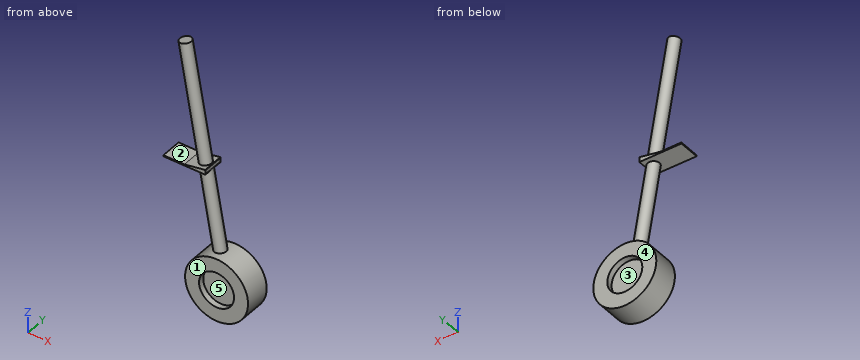
from build123d import *

# Parameters (mm, degrees)
F0_W      = 180
F0_H      = 90
F1_DEPTH  = 5
F3_DEPTH  = 90
F4_R      = 25
F5_DEPTH  = 495
F6_DEPTH  = 500
F9_R      = 135
F10_DEPTH = 55
F11_R     = 75
F12_DEPTH = 25
F13_R     = 75
F14_DEPTH = 25


with BuildPart() as f1:
    # F0 (on Top) → F1 (new body)
    with BuildSketch(Plane.XY):
        Rectangle(F0_W, F0_H)
    extrude(amount=F1_DEPTH)

    # F2 (on face) → F3 (join)
    with BuildSketch(Plane.XZ.offset(45)):
        Polygon((88.6326977711, 20.62833599), (0, 5), (28.4956841358, 5), (89.5009386594, 15.704297225), align=None)
        Polygon((89.5009386594, 15.704297225), (28.4956841358, 5), (90, 5), align=None)
    extrude(amount=-F3_DEPTH)

    # F4 (on face) → F5 (join)
    with BuildSketch(Plane(origin=(-0.8550503583, 0, 4.849231552), x_dir=(0.984807753, 0, 0.1736481777), z_dir=(-0.1736481777, 0, 0.984807753))):
        with Locations((60.8682408883, 0)):
            Circle(F4_R)
    extrude(amount=-F5_DEPTH)

    # F4 (on face) → F6 (join)
    with BuildSketch(Plane(origin=(-0.8550503583, 0, 4.849231552), x_dir=(0.984807753, 0, 0.1736481777), z_dir=(-0.1736481777, 0, 0.984807753))):
        with Locations((60.8682408883, 0)):
            Circle(F4_R)
    extrude(amount=F6_DEPTH)

    # F9 (on line) → F10 (join, symmetric)
    with BuildSketch(Plane(origin=(0, 0, 0), x_dir=(-1, 0, 0), z_dir=(0, 1, 0))):
        with Locations((-145.0443131259, -472.060947081)):
            Circle(F9_R)
    extrude(amount=F10_DEPTH, both=True)

    # F11 (on face) → F12 (cut)
    with BuildSketch(Plane.XZ.offset(55)):
        with Locations((145.0443131259, -472.060947081)):
            Circle(F11_R)
    extrude(amount=-F12_DEPTH, mode=Mode.SUBTRACT)

    # F13 (on face) → F14 (cut)
    with BuildSketch(Plane(origin=(0, 55, 0), x_dir=(-1, 0, 0), z_dir=(0, 1, 0))):
        with Locations((-145.0443131259, -472.060947081)):
            Circle(F13_R)
    extrude(amount=-F14_DEPTH, mode=Mode.SUBTRACT)


solid = f1.part
The model under review builds one solid part; all positions refer to its coordinate system, in mm. Face numbers are marked on the shaded views. A direction names the side the tool comes from. Round coordinates to 2 decimals unless told otherwise and drop trailing zeros. Write each loop counter-clockwise with the first axis right and the second up, starting at its lowest first coordinate (ties: lowest second). Pieces come first, ordered by that corner, then holes. Notation, with made-up numbers: (-10, -37.5) -> (-1, -37.5) arc R27 cw to (-1, -10.5) -> close; hole circle Ø9 at (-8.5, -34.75). An arc over 180 degrees is marked (long way). Answer as a JSON object with one key per item and string values.
1. We need section C-C on x = 204.5. State the section outline as (y, z) points, and give its area (3 significant figures).
Results found:
{"outline": "(-55, -593.26) -> (55, -593.26) -> (55, -517.78) -> (30, -517.78) -> (30, -426.34) -> (55, -426.34) -> (55, -350.86) -> (-55, -350.86) -> (-55, -426.34) -> (-30, -426.34) -> (-30, -517.78) -> (-55, -517.78) -> close", "area": "22,100 mm^2"}
2. We need section A-A on y = -13.5. State the section outline as (x, z) points, and give its area (3 significant figures).
Results found:
{"outline": "(-90, 0) -> (40.44, 0) -> (101.17, -344.39) arc R135 ccw (long way) to (142.61, -337.08) -> (83.17, 0) -> (90, 0) -> (90, 5) -> (89.5, 15.7) -> (88.63, 20.63) -> (79.81, 19.07) -> (-7.01, 511.48) -> (-48.46, 504.17) -> (38.37, 11.77) -> (0, 5) -> (-90, 5) -> close", "area": "94,400 mm^2"}
3. The part is to be moulded in two halves that separate along X. For the marked faces 3, 4 and 5, say which applies: pulls with the +X half, pulls with the -X half, needs draft (parallel to the pull), parting line crosses it, or undercut.
Results found:
{"face 3": "undercut", "face 4": "needs draft", "face 5": "undercut"}
4. Clearance check with flat-ended pins moving along their axes: pin 1 (1 mm diameter, centred on x = 204.5, y = 0, fed in from +Z); pin 2 (5.5 mm diameter, centred on y = 16, z = 2, fed in from +X); pin 3 (10.5 mm diameter, centred on x = 25.5, z = 11.5, fed in from +Y). State where each tip first meets the part, or that it passes through.
Results found:
{"pin 1": "stops at z = -350.61", "pin 2": "stops at x = 90", "pin 3": "stops at y = 45"}
5. To check wall thickness, follow line 1 along Z through (x, y) = (187, 37); line 2 along X through (y, z) = (-14.5, 376.5); line 3 along X through (y, z) = (-11, -110.5). State the ranges of each line that lie inside material, in increasing order.
Results found:
{"line 1": "z = -600.38 to -534.23, -409.89 to -343.75", "line 2": "x = -25.26 to 16.1", "line 3": "x = 58.5 to 104.09"}
6. We need section B-B on x = 159. State the section outline as (y, z) points.
Results found:
{"outline": "(-55, -606.34) -> (55, -606.34) -> (55, -545.75) -> (30, -545.75) -> (30, -398.37) -> (55, -398.37) -> (55, -337.78) -> (-55, -337.78) -> (-55, -398.37) -> (-30, -398.37) -> (-30, -545.75) -> (-55, -545.75) -> close"}
7. Machinability: for the marked faces 1 and 2, which of the approach directions +Z, -Z, +X, -X, +Y, -Y give a long, thin tool a straight path to every point of the face, cutting with its end or side? Answer none if there is none.
Results found:
{"face 1": "+Z, -Z, +X, -X, -Y", "face 2": "-X, +Y, -Y"}
